Part model, mm, in its own coordinate system. A direction names the side the tool comes from. Give positions to 0.01 mm unless a question says otherwise; leave off trailing zeros. Write each loop counter-clockwise with the first axis right and the second up, starting at its lowest first coordinate (ties: lowest second). Pieces come first, ordered by that corner, then holes. Notation, with made-up numbers: (56.5, 27.25) - (74.5, 27.25) arc R7 cw to (74.5, 36.25) - close; hole circle Ø2 at (-12, 32). An arc over 180 degrees is marked (long way). Answer as a JSON object with one key per item and string values. Group by question number.
Autodesk Inventor part; units mm, degrees
ref_plane "YZ Plane" through (0, 0, 0) normal (1, 0, 0) x (0, 1, 0)
ref_plane "XZ Plane" through (0, 0, 0) normal (0, 1, 0) x (-1, 0, 0)
ref_plane "XY Plane" through (0, 0, 0) normal (0, 0, 1) x (1, 0, 0)
sketch "Sketch1" plane through (0, 0, 0) normal (0, 1, 0) x (-1, 0, 0)
  line L0 (0, 0) -> (50.8, 0)
  line L1 (50.8, 0) -> (50.8, -76.2)
  line L2 (50.8, -76.2) -> (0, -76.2)
  line L3 (0, -76.2) -> (0, 0)
  dimension "d0" = 50.8
  dimension "d1" = 76.2
extrude "Extrusion1" add sketch "Sketch1" along normal blind 13.97
sketch "Sketch6" plane through (0, 13.97, 0) normal (0, 1, 0) x (1, 0, 0)
  point P0 (0, 0)
sketch "Sketch7" plane through (0, 13.97, 0) normal (0, 1, 0) x (1, 0, 0)
  point P0 (0, 0)
sketch "Sketch8" plane through (0, 13.97, 0) normal (0, 1, 0) x (1, 0, 0)
  circle A0 centre (-25.4, 38.1) radius 22.86
  circle A1 centre (-25.4, 38.1) radius 19.05
  point P0 (0, 0)
  dimension "d30" = 45.72
  dimension "d31" = 38.1
extrude "Extrusion15" add sketch "Sketch8" along normal blind 3.81
sketch "Sketch9" plane through (-25.4, 13.97, -38.1) normal (0, 1, 0) x (1, 0, 0)
  line L0 (-8.6694, 8.1535) -> (3.6792, 8.1535)
  line L1 (3.6792, 8.1535) -> (3.6792, 9.8977)
  line L2 (3.6792, 9.8977) -> (5.4931, 11.4325)
  line L3 (5.4931, 11.4325) -> (5.4931, 0.0971)
  line L4 (-8.6694, 8.1535) -> (-8.6694, 0.0971)
  line L5 (-8.6694, -7.9593) -> (3.6792, -7.9593)
  line L6 (3.6792, -7.9593) -> (3.6792, -9.7035)
  line L7 (3.6792, -9.7035) -> (5.4931, -11.2383)
  line L8 (5.4931, -11.2383) -> (5.4931, 0.0971)
  line L9 (-8.6694, -7.9593) -> (-8.6694, 0.0971)
  line L10 (8.2546, 0.0971) -> (8.2546, -14.3778)
  line L11 (8.2546, -14.3778) -> (2.1623, -14.3778)
  line L12 (2.1623, -14.3778) -> (2.1623, -11.2383)
  line L13 (2.1623, -11.2383) -> (-10.3102, -11.2383)
  line L14 (-10.3102, -11.2383) -> (-10.3102, 0.0971)
  line L15 (8.2546, 0.0971) -> (8.2546, 14.572)
  line L16 (8.2546, 14.572) -> (2.1623, 14.572)
  line L17 (2.1623, 14.572) -> (2.1623, 11.4325)
  line L18 (2.1623, 11.4325) -> (-10.3102, 11.4325)
  line L19 (-10.3102, 11.4325) -> (-10.3102, 0.0971)
  line L20 (-12.1685, 0.0971) -> (-12.1685, -3.512)
  line L21 (-12.1685, -3.512) -> (-10.3102, -3.512)
  line L22 (-10.3102, -3.512) -> (-10.3102, 0.0971)
  line L23 (-12.1685, 0.0971) -> (-12.1685, 3.7061)
  line L24 (-12.1685, 3.7061) -> (-10.3102, 3.7061)
  line L25 (10.4745, 0.0971) -> (10.4745, -3.512)
  line L26 (10.4745, -3.512) -> (8.2546, -3.512)
  line L27 (8.2546, -3.512) -> (8.2546, 0.0971)
  line L28 (10.4745, 0.0971) -> (10.4745, 3.7061)
  line L29 (10.4745, 3.7061) -> (8.2546, 3.7061)
  point P0 (25.4, -38.1)
  point P1 (8.2546, -3.512)
  point P2 (8.2546, 3.7061)
  point P3 (-10.3102, 3.7061)
  point P4 (-10.3102, -3.512)
extrude "Extrusion16" add sketch "Sketch9" along normal blind 5.08
properties part number "CNC#2 FInal"
1) Saw through at B-B (z = -38.1). List the corners of the cut face in (x, y).
2) Saw through at C-C (x = -25.4). List the corners of the cut face in (y, z).
3) Drill centre lines: line 1 along X through (y, z) = (16.5, -38.1); line 2 along Z through (x, y) = (-25.4, 15.1); line 3 along Y through (x, z) = (-47.5, -72). Where is each one in solid material? Low to high. Write a range as from..to.
4) Drop flat-ended pins along their axis: P1, Ø3, axis at x = -10.5, z = -12, coming from the +Y side; P2, Ø2, axis at x = -36.5, y = 16.5, coming from the -Z side; P3, Ø1.5, axis at x = -18.5, y = 17.5, coming from the +Z side. Give the stop position or say it passes through.
5) Saw through at A-A (y = 16.5). List the corners of the cut face in (x, z).
6) Which spindle directions (+Z, -Z, +X, -X, +Y, -Y) get a long thin tool onto all of the face, cutting with end or side? Do faces 1 (the flat face through (-19.6, 19.05, -37.2)), 2 (the flat face through (-37, 16, -41.806)). Say none if no direction does.
7) Two-plate mould, pull along X, no slides. Class faces 3 (the flat face through (-26, 7, -76.2)), 4 (the cylindrical face through (-30.356, 15.848, -60.416)), 5 (the flat face through (-21.721, 16, -29)): +X half, -X half, draft (parallel to the pull), parting line (faces both ways), or undercut.
8) Saw through at D-D (x = -5.5). List the corners of the cut face in (y, z), and give its area (3 significant figures).
Checks:
{
 "1": {"outline": "(-50.8, 0) - (0, 0) - (0, 13.97) - (-2.54, 13.97) - (-2.54, 17.78) - (-6.35, 17.78) - (-6.35, 13.97) - (-14.93, 13.97) - (-14.93, 19.05) - (-19.91, 19.05) - (-19.91, 13.97) - (-34.07, 13.97) - (-34.07, 19.05) - (-37.57, 19.05) - (-37.57, 13.97) - (-44.45, 13.97) - (-44.45, 17.78) - (-48.26, 17.78) - (-48.26, 13.97) - (-50.8, 13.97) - close"},
 "2": {"outline": "(0, -76.2) - (13.97, -76.2) - (13.97, -60.96) - (17.78, -60.96) - (17.78, -57.15) - (13.97, -57.15) - (13.97, -49.53) - (19.05, -49.53) - (19.05, -46.25) - (13.97, -46.25) - (13.97, -30.14) - (19.05, -30.14) - (19.05, -26.86) - (13.97, -26.86) - (13.97, -19.05) - (17.78, -19.05) - (17.78, -15.24) - (13.97, -15.24) - (13.97, 0) - (0, 0) - close"},
 "3": {"line 1": "-48.26..-44.45, -37.57..-34.07, -19.91..-14.93, -6.35..-2.54", "line 2": "-60.96..-57.15, -49.53..-46.25, -30.14..-26.86, -19.05..-15.24", "line 3": "0..13.97"},
 "4": {"P1": "y = 13.97", "P2": "z = -58.61", "P3": "z = -16.08"},
 "5": {"outline": "circle Ø45.72 at (-25.4, -38.1); (-37.57, -41.81) - (-35.71, -41.81) - (-35.71, -49.53) - (-23.24, -49.53) - (-23.24, -52.67) - (-17.15, -52.67) - (-17.15, -41.81) - (-14.93, -41.81) - (-14.93, -34.59) - (-17.15, -34.59) - (-17.15, -23.72) - (-23.24, -23.72) - (-23.24, -26.86) - (-35.71, -26.86) - (-35.71, -34.59) - (-37.57, -34.59) - close; hole circle Ø38.1 at (-25.4, -38.1); hole (-34.07, -46.25) - (-21.72, -46.25) - (-21.72, -48) - (-19.91, -49.53) - (-19.91, -26.86) - (-21.72, -28.4) - (-21.72, -30.14) - (-34.07, -30.14) - close"},
 "6": {"face 1": "+Z, -Z, +X, -X, +Y", "face 2": "+Y"},
 "7": {"face 3": "draft", "face 4": "parting line", "face 5": "undercut"},
 "8": {"outline": "(0, -76.2) - (13.97, -76.2) - (13.97, -49.35) - (17.78, -49.35) - (17.78, -26.85) - (13.97, -26.85) - (13.97, 0) - (0, 0) - close", "area": "1,150 mm2"}
}
